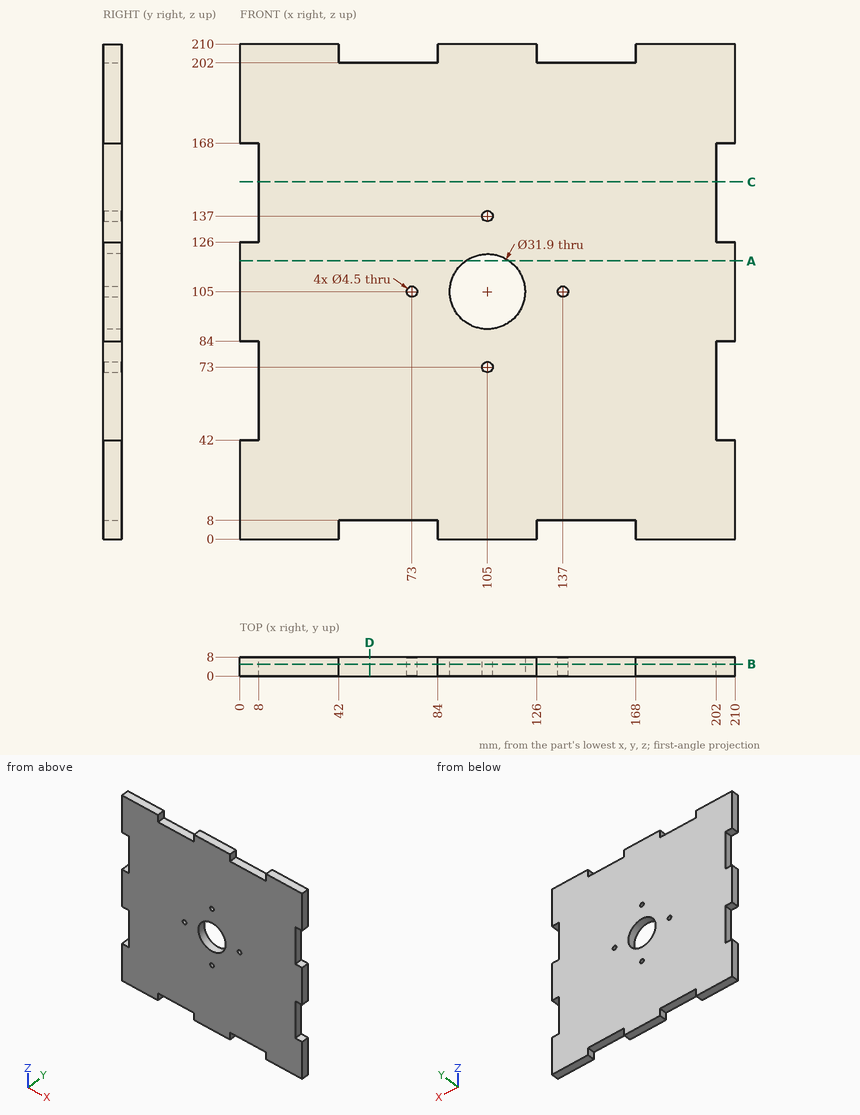
Geometry: see drawing. Coordinates: mm, zero at the bounding-box minimum. Coordinates: 2 decimals unless noted, no trailing zeros. Loops run counter-clockwise (first coordinate to the right, second up) from the corner with the lowest first, then second, coordinate; pieces in that order, holes last.
Q1. Cut plane A-A (z = 118). Output: boundary loops of the cut face in (x, y).
Q2. Cut plane D-D (x = 55). Output: boundary loops of the cut face in (y, z), then the cut area to 3 significant figures.
Q3. Contact query for flat-ended pins moving along their axis: pin 1 (4 mm diameter, centred on y = 5, z = 61, fed in from +X); pin 2 (3.5 mm diameter, centred on x = 105, z = 73, fed in from +Y); pin 3 (4 mm diameter, centred on x = 70.5, y = 4.5, fed in from -Z). Output: stop coordinate, or through.
Q4. Cut plane B-B (y = 5). Give the number of separate pieces and of enclosed holes in the cut face, then the cut area to 3 significant figures.
Q5. Cut plane C-C (z = 151.5). Output: boundary loops of the cut face in (x, y), then the cut area to 3 significant figures.
Q6. Material intervals for line 1 (Z direction, x = 105, y = 4.75); line 2 (X direction, y = 4.5, z = 137); line 3 (Z direction, x = 131.5, y = 2.5), sorted ascending.
Working result:
1. outline: (0, 0) - (95.76, 0) - (95.76, 8) - (0, 8) - close; (114.24, 0) - (210, 0) - (210, 8) - (114.24, 8) - close
2. outline: (0, 8) - (8, 8) - (8, 202) - (0, 202) - close
2. area: 1,550 mm2
3. pin 1: stops at x = 202
3. pin 2: passes through
3. pin 3: stops at z = 8
4. separate pieces: 1
4. enclosed holes: 5
4. area: 40,500 mm2
5. outline: (8, 0) - (202, 0) - (202, 8) - (8, 8) - close
5. area: 1,550 mm2
6. line 1: z = 0 to 70.75, 75.25 to 89.05, 120.95 to 134.75, 139.25 to 210
6. line 2: x = 8 to 102.75, 107.25 to 202
6. line 3: z = 8 to 202
